```python
from build123d import *

# Parameters (mm, degrees)
ESQUISSE1_W             = 180
ESQUISSE1_H             = 410
ESQUISSE1_W_2           = 138
ESQUISSE1_H_2           = 300
BOSS_EXTRU_1_DEPTH      = 20
CONG_1_R                = 3
ESQUISSE2_R             = 2
ENL_V_MAT_EXTRU_1_DEPTH = 362.939221417
ESQUISSE3_R             = 1.5
ENL_V_MAT_EXTRU_2_DEPTH = 225.77766793
ESQUISSE4_R             = 3.5
ENL_V_MAT_EXTRU_3_DEPTH = 274.541587332
ESQUISSE5_W             = 99
ESQUISSE5_H             = 12
BOSS_EXTRU_2_DEPTH      = 18
ESQUISSE12_W            = 3
ESQUISSE12_H            = 3
BOSS_EXTRU_5_DEPTH      = 99
ESQUISSE13_W            = 6
ESQUISSE13_H            = 6.6095607
ENL_V_MAT_EXTRU_5_DEPTH = 99
ENL_V_MAT_EXTRU_6_DEPTH = 6.6095607
ESQUISSE15_R            = 2
ENL_V_MAT_EXTRU_7_DEPTH = 373.643309543


with BuildPart() as part:
    # Esquisse1 → Boss.-Extru.1 (new body)
    with BuildSketch(Plane.XY):
        Rectangle(ESQUISSE1_W, ESQUISSE1_H)
        with Locations((0, -5)):
            Rectangle(ESQUISSE1_W_2, ESQUISSE1_H_2, mode=Mode.SUBTRACT)
    extrude(amount=BOSS_EXTRU_1_DEPTH)

    # Congé1
    cong_1_edges = [part.edges().sort_by_distance(p)[0] for p in [
        (90, 0, 20),
        (-69, -5, 0),
        (-69, 145, 10),
        (0, -155, 0),
        (-69, -155, 10),
        (69, -5, 0),
        (69, -155, 10),
        (0, 145, 0),
        (69, 145, 10),
        (-69, -5, 20),
        (0, 205, 20),
        (0, -155, 20),
        (69, -5, 20),
        (0, 145, 20),
        (-90, 0, 20),
        (0, 205, 0),
        (90, 0, 0),
        (0, -205, 0),
        (-90, 0, 0),
        (90, -205, 10),
        (-90, -205, 10),
        (0, -205, 20),
    ]]
    fillet(cong_1_edges, radius=CONG_1_R)

    # Esquisse2 → Enlèv. mat.-Extru.1 (cut, through all)
    with BuildSketch(Plane.XZ.offset(-145)):
        with Locations((-30, 10)):
            Circle(ESQUISSE2_R)
        with Locations(Location((30, 10, 0), (0, 0, 180))):
            Circle(ESQUISSE2_R)
    extrude(amount=-ENL_V_MAT_EXTRU_1_DEPTH, mode=Mode.SUBTRACT)

    # Esquisse3 → Enlèv. mat.-Extru.2 (cut, through all)
    with BuildSketch(Plane.XY.offset(20)):
        with Locations((-79.79859846, 111.493173655)):
            Circle(ESQUISSE3_R)
        with Locations(Location((79.79859846, 111.493173655, 0), (0, 0, 180))):
            Circle(ESQUISSE3_R)
    extrude(amount=-ENL_V_MAT_EXTRU_2_DEPTH, mode=Mode.SUBTRACT)

    # Esquisse4 → Enlèv. mat.-Extru.3 (cut, through all)
    with BuildSketch(Plane.ZY.offset(90)):
        with Locations(Location((9.507126216, -194.754948591, 0), (0, 0, 270))):
            Circle(ESQUISSE4_R)
    extrude(amount=-ENL_V_MAT_EXTRU_3_DEPTH, mode=Mode.SUBTRACT)

    # Esquisse5 → Boss.-Extru.2 (add)
    with BuildSketch(Plane.XY.offset(20)):
        with Locations((0, -154)):
            Rectangle(ESQUISSE5_W, ESQUISSE5_H)
    extrude(amount=BOSS_EXTRU_2_DEPTH)

    # Esquisse12 → Boss.-Extru.5 (add)
    with BuildSketch(Plane.ZY.offset(49.5)):
        with Locations((36.5, -146.5)):
            Rectangle(ESQUISSE12_W, ESQUISSE12_H)
    extrude(amount=-BOSS_EXTRU_5_DEPTH)

    # Esquisse13 → Enlèv. mat.-Extru.5 (cut)
    with BuildSketch(Plane.ZY.offset(49.5)):
        with Locations((32, -151.30478035)):
            Rectangle(ESQUISSE13_W, ESQUISSE13_H)
    extrude(amount=-ENL_V_MAT_EXTRU_5_DEPTH, mode=Mode.SUBTRACT)

    # Esquisse14 → Enlèv. mat.-Extru.6 (cut)
    with BuildSketch(Plane(origin=(0, -148, 0), x_dir=(1, 0, 0), z_dir=(0, 1, 0))):
        with BuildLine():
            Line((-47.5, -29), (-47.5, -22))
            Line((-47.5, -22), (-1, -22))
            Line((-1, -22), (-1, -24.7))
            ThreePointArc((-1, -24.7), (-0.912132034, -24.912132034), (-0.7, -25))
            Line((-0.7, -25), (0.7, -25))
            ThreePointArc((0.7, -25), (0.912132034, -24.912132034), (1, -24.7))
            Line((1, -24.7), (1, -22))
            Line((1, -22), (47.5, -22))
            Line((47.5, -22), (47.5, -29))
            Line((47.5, -29), (-47.5, -29))
        make_face()
    extrude(amount=-ENL_V_MAT_EXTRU_6_DEPTH, mode=Mode.SUBTRACT)

    # Esquisse15 → Enlèv. mat.-Extru.7 (cut, through all)
    with BuildSketch(Plane(origin=(0, -154.6095607, 0), x_dir=(1, 0, 0), z_dir=(0, 1, 0))):
        with Locations(Location((-23.5, -25, 0), (0, 0, 180))):
            Circle(ESQUISSE15_R)
        with Locations(Location((23.5, -25, 0), (0, 0, 270))):
            Circle(ESQUISSE15_R)
    extrude(amount=-ENL_V_MAT_EXTRU_7_DEPTH, mode=Mode.SUBTRACT)


solid = part.part
```
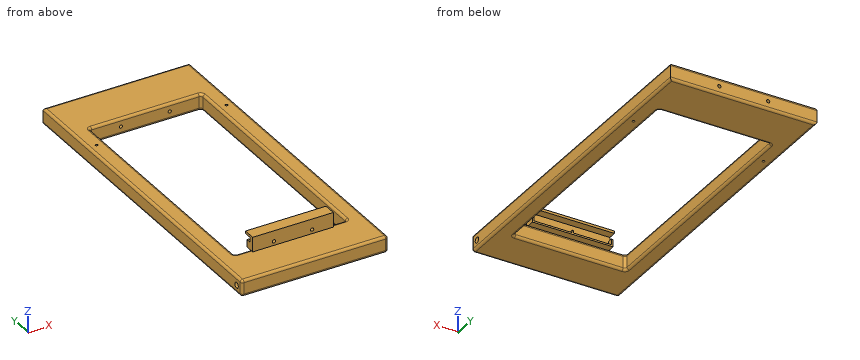
Can you work these out from the model? Positions are in its coordinate system, mm. Give positions to 0.01 mm unless a question says otherwise; leave off trailing zeros. Order: outer loops, then holes, each group sorted by start corner. A loop starts at its lowest first (then second) coordinate and runs counter-clockwise, first axis right, second up. Notation, with made-up numbers: (-21.5, 22.25) - (-10.5, 22.25) arc R31 ccw to (-10.5, 49.25) - close; hole circle Ø1 at (80, 58.25). An arc over 180 degrees is marked (long way). Use a Markdown table: item, result. Add a question column.
Q1. If we section it at B-B on x = -55: Write out the boundary of the cut face in (y, z), plus the area to 3 significant figures.
Q2. If we section it at C-C on y = 175: Write out the boundary of the cut face in (x, z).
Q3. Please list where these lines run through material, in increasing order: line 1 along Y through (x, z) = (19, 14.5); line 2 along X through (y, z) = (38.5, 11); line 3 along Y through (x, z) = (-47, 12.5).
Q4. If we section it at A-A on y = -64: Write out the boundary of the cut face in (x, z), plus the area to 3 significant figures.
Q5. I'm going to push flat-ended pins straight in: pin 1 (8 mm diameter, centred on x = 18, y = -152.5, fed in from -Z); pin 2 (2.5 mm diameter, centred on x = 23.5, z = 25, fed in from +Y); pin 3 (3 mm diameter, centred on x = -3, z = 24.5, fed in from -Y); pin 4 (4 mm diameter, centred on x = 8, z = 28, fed in from +Y). Where does each tip first touch, or does it pass through?
Answers follow:
| question | item | result |
|---|---|---|
| 1 | outline | (-205, 3) arc R3 ccw to (-202, 0) - (-158, 0) arc R3 ccw to (-155, 3) - (-155, 17) arc R3 ccw to (-158, 20) - (-202, 20) arc R3 ccw to (-205, 17) - close; (145, 3) arc R3 ccw to (148, 0) - (202, 0) arc R3 ccw to (205, 3) - (205, 17) arc R3 ccw to (202, 20) - (148, 20) arc R3 ccw to (145, 17) - close; hole circle Ø7 at (-194.75, 9.51) |
| 1 | area | 2,150 mm^2 |
| 2 | outline | (-90, 3) arc R3 ccw to (-87, 0) - (87, 0) arc R3 ccw to (90, 3) - (90, 17) arc R3 ccw to (87, 20) - (-87, 20) arc R3 ccw to (-90, 17) - close; hole circle Ø4 at (-30, 10); hole circle Ø4 at (30, 10) |
| 3 | line 1 | y = -205 to -155, 145 to 205 |
| 3 | line 2 | x = -90 to -69, 69 to 90 |
| 3 | line 3 | y = -205 to -196.57, -192.94 to -155, 145 to 205 |
| 4 | outline | (-90, 3) arc R3 ccw to (-87, 0) - (-72, 0) arc R3 ccw to (-69, 3) - (-69, 17) arc R3 ccw to (-72, 20) - (-87, 20) arc R3 ccw to (-90, 17) - close; (69, 3) arc R3 ccw to (72, 0) - (87, 0) arc R3 ccw to (90, 3) - (90, 17) arc R3 ccw to (87, 20) - (72, 20) arc R3 ccw to (69, 17) - close |
| 4 | area | 825 mm^2 |
| 5 | pin 1 | stops at z = 0.4 |
| 5 | pin 2 | passes through |
| 5 | pin 3 | stops at y = -160 |
| 5 | pin 4 | stops at y = -154.61 |
